```python
from build123d import *

# Parameters (mm, degrees)
ESQUISSE1_W             = 70
ESQUISSE1_H             = 28
BOSS_EXTRU_1_DEPTH      = 11
ESQUISSE2_R             = 1.5
ENL_V_MAT_EXTRU_1_DEPTH = 29
ESQUISSE3_R             = 6.8
ENL_V_MAT_EXTRU_2_DEPTH = 12
ESQUISSE4_R             = 12
ENL_V_MAT_EXTRU_3_DEPTH = 4
ESQUISSE5_W             = 10
ESQUISSE5_H             = 20
ENL_V_MAT_EXTRU_4_DEPTH = 12
ESQUISSE6_W             = 10
ESQUISSE6_H             = 20
ENL_V_MAT_EXTRU_5_DEPTH = 12


with BuildPart() as part:
    # Esquisse1 → Boss.-Extru.1 (new body)
    with BuildSketch(Plane.XY):
        Rectangle(ESQUISSE1_W, ESQUISSE1_H)
    extrude(amount=BOSS_EXTRU_1_DEPTH)

    # Esquisse2 → Enlèv. mat.-Extru.1 (cut, through all)
    with BuildSketch(Plane(origin=(0, 14, 0), x_dir=(1, 0, 0), z_dir=(0, 1, 0))):
        with Locations((30, -2.5)):
            Circle(ESQUISSE2_R)
        with Locations((-30, -2.5)):
            Circle(ESQUISSE2_R)
    extrude(amount=-ENL_V_MAT_EXTRU_1_DEPTH, mode=Mode.SUBTRACT)

    # Esquisse3 → Enlèv. mat.-Extru.2 (cut, through all)
    with BuildSketch(Plane.XY.offset(11)):
        Circle(ESQUISSE3_R)
    extrude(amount=-ENL_V_MAT_EXTRU_2_DEPTH, mode=Mode.SUBTRACT)

    # Esquisse4 → Enlèv. mat.-Extru.3 (cut)
    with BuildSketch(Plane.XY.offset(11)):
        Circle(ESQUISSE4_R)
    extrude(amount=-ENL_V_MAT_EXTRU_3_DEPTH, mode=Mode.SUBTRACT)

    # Esquisse5 → Enlèv. mat.-Extru.4 (cut, through all)
    with BuildSketch(Plane.XY.offset(11)):
        with Locations((-30, 0)):
            Rectangle(ESQUISSE5_W, ESQUISSE5_H)
    extrude(amount=-ENL_V_MAT_EXTRU_4_DEPTH, mode=Mode.SUBTRACT)

    # Esquisse6 → Enlèv. mat.-Extru.5 (cut, through all)
    with BuildSketch(Plane.XY.offset(11)):
        with Locations((30, 0)):
            Rectangle(ESQUISSE6_W, ESQUISSE6_H)
    extrude(amount=-ENL_V_MAT_EXTRU_5_DEPTH, mode=Mode.SUBTRACT)


solid = part.part
```
For this review, take the finished solid that the model builds, in its own axes (mm). A direction names the side the tool comes from. Give positions to 0.01 mm unless a question says otherwise; leave off trailing zeros. Loops run counter-clockwise (first coordinate to the right, second up) from the corner with the lowest first, then second, coordinate; pieces in that order, holes last. Notation, with made-up numbers: M 64.25,-33 L 110.25,-33 A17 ccw 110.25,-26 Z; hole C -31,0.5 d7. An arc over 180 degrees is marked long. One line per item, written item: value. Start each with the question number.
Q1. For L1, parallel to X at y = 11.65, z = 2.5; L2, parallel to Y at x = -30, z = 6.75; L3, parallel to Z at x = 30, y = -11.45, list the stretches that pass through material, from the lowest coordinate up.
Q2. Machinability: for faces 1 (the face through (-25, 0, 6)), 2 (the face through (30, 10, 6)), 3 (the face through (-11.99, 0.53, 9.03)), which of the approach directions +Z, -Z, +X, -X, +Y, -Y give a long, thin tool a straight path to every point of the face, cutting with its end or side? Answer none if there is none.
Q3. Add section C-C (x = 0). Give the boundary of the cut face in (y, z), and give its area (3 significant figures).
Q4. Add section B-B (y = 0). Give the boundary of the cut face in (x, z), and give its area (3 significant figures).
Q5. Add section A-A (z = 2.5). Count the separate pieces of the cut face and the enclosed holes in it, and give its area (3 significant figures).
Q6. Draft analysis for pull direction X (two halves, no side actions). For faces 4 (the face through (0, -14, 5)), 5 (the face through (35, -12, 5)), 6 (the face through (-31.5, 12.03, 2.43)), 7 (the face through (-35, -12, 5)), state which applies: released by +X, released by -X, zero draft, split by the parting line, or undercut.
Q7. Add section D-D (x = -30). Give the boundary of the cut face in (y, z), and give its area (3 significant figures).
Q8. Clearance check with flat-ended pins moving along their axes: pin 1 Ø3.5 at (x, z) = (-30, 2.5) entering from +Y; pin 2 Ø12 at (x, y) = (-5, -3) entering from +Z. State where each tip first meets the part, or that it passes through.
Reply:
1. L1: -35 to -31.5, -28.5 to 28.5, 31.5 to 35
1. L2: -14 to -10, 10 to 14
1. L3: 0 to 1, 4 to 11
2. face 1: +Z, -Z, -X
2. face 2: +Z, -Z, +X
2. face 3: +Z
3. outline: M -14,0 L -6.8,0 L -6.8,7 L -12,7 L -12,11 L -14,11 Z; M 6.8,0 L 14,0 L 14,11 L 12,11 L 12,7 L 6.8,7 Z
3. area: 117 mm²
4. outline: M -25,0 L -6.8,0 L -6.8,7 L -12,7 L -12,11 L -25,11 Z; M 6.8,0 L 25,0 L 25,11 L 12,11 L 12,7 L 6.8,7 Z
4. area: 359 mm²
5. separate pieces: 5
5. enclosed holes: 1
5. area: 1,370 mm²
6. face 4: zero draft
6. face 5: released by +X
6. face 6: undercut
6. face 7: released by -X
7. outline: M -14,0 L -10,0 L -10,1 L -14,1 Z; M -14,4 L -10,4 L -10,11 L -14,11 Z; M 10,0 L 14,0 L 14,1 L 10,1 Z; M 10,4 L 14,4 L 14,11 L 10,11 Z
7. area: 64.0 mm²
8. pin 1: y = 14
8. pin 2: z = 7
